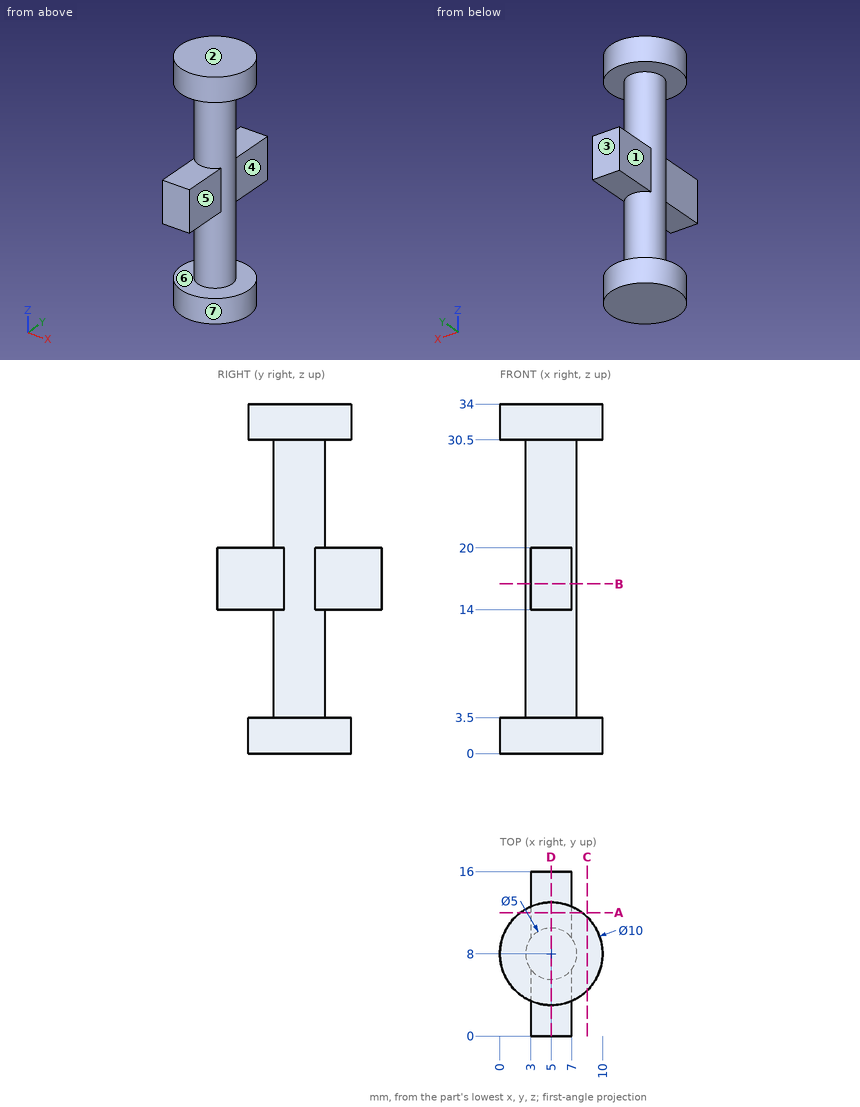
Geometry: see drawing. Coordinates: mm, zero at the bounding-box minimum. A direction names the side the tool comes from. Give positions to 0.01 mm unless a question says otherwise; leave off trailing zeros. Order: outer loops, then holes, each group sorted by start corner. A loop starts at its lowest first (then second) coordinate and runs counter-clockwise, first axis right, second up. Notation, with made-up numbers: (41.5, 11) -> (69.5, 11) arc R32 cw to (69.5, 40) -> close; hole circle Ø11 at (28, 32). An arc over 180 degrees is marked (long way). Write item = value, one per line.
Q1. Pull-direction query (Z, two-part tool) for the marked faces 1, 2, 3 and 4; classes: released by +Z, released by -Z, zero draft, split by the parting line, or undercut.
Data:
face_1 = undercut
face_2 = released by +Z
face_3 = zero draft
face_4 = undercut
Q2. Material intervals for line 1 (Z direction, x = 4.75, y = 3.5); line 2 (X direction, y = 13.75, z = 15.5); line 3 (Z direction, x = 7.25, y = 5), sorted ascending. Write a range as from..to.
Data:
line_1 = 0..3.5, 14..20, 30.5..34
line_2 = 3..7
line_3 = 0..3.5, 30.5..34
Q3. Cut plane C-C, the plane x = 8.5. Output: boundary loops of the cut face in (y, z).
Data:
outline = (4.43, 0) -> (11.57, 0) -> (11.57, 3.5) -> (4.43, 3.5) -> close; (4.43, 30.5) -> (11.57, 30.5) -> (11.57, 34) -> (4.43, 34) -> close
Q4. Cut plane B-B, the plane z = 16.5. Output: boundary loops of the cut face in (x, y), and give its area (3 significant figures).
Data:
outline = (3, 0) -> (7, 0) -> (7, 6.5) arc R2.5 ccw to (7, 9.5) -> (7, 16) -> (3, 16) -> (3, 9.5) arc R2.5 ccw to (3, 6.5) -> close
area = 66.0 mm^2
Q5. Set-up query: the marked faces 5, 6 and 7. Return all of +Z, -Z, +X, -X, +Y, -Y with unobstructed straight access to the full face (end or side cutting, diameter ignored); none if empty.
Data:
face_5 = +X, -Y
face_6 = none
face_7 = -Z
Q6. Cut plane A-A, the plane y = 12. Output: boundary loops of the cut face in (x, z), and give its area (3 significant figures).
Data:
outline = (2, 0) -> (8, 0) -> (8, 3.5) -> (2, 3.5) -> close; (2, 30.5) -> (8, 30.5) -> (8, 34) -> (2, 34) -> close; (3, 14) -> (7, 14) -> (7, 20) -> (3, 20) -> close
area = 66.0 mm^2
Q7. Cut plane D-D, the plane x = 5. Output: boundary loops of the cut face in (y, z), and give its area (3 significant figures).
Data:
outline = (0, 14) -> (5.5, 14) -> (5.5, 3.5) -> (3, 3.5) -> (3, 0) -> (13, 0) -> (13, 3.5) -> (10.5, 3.5) -> (10.5, 14) -> (16, 14) -> (16, 20) -> (10.5, 20) -> (10.5, 30.5) -> (13, 30.5) -> (13, 34) -> (3, 34) -> (3, 30.5) -> (5.5, 30.5) -> (5.5, 20) -> (0, 20) -> close
area = 271 mm^2
Q8. Pin query (flat end, axial travel): pin 1 (6 mm diameter, centred on x = 5.5, z = 8, fed in from -Y); pin 2 (3 mm diameter, centred on x = 5, y = 2.5, fed in from -Z); pin 3 (3 mm diameter, centred on y = 2, z = 16, fed in from -X); pin 4 (3 mm diameter, centred on y = 12.5, z = 16, fed in from +X). Return the tip coordinate at first contact, or that it passes through.
Data:
pin_1 = 5.5
pin_2 = 0
pin_3 = 3
pin_4 = 7
